Read the model definition and answer for the solid it produces. Units are mm, in the model's axes. Face numbers are marked on the shaded views. Round coordinates to 2 decimals unless told otherwise and drop trailing zeros. Write each loop counter-clockwise with the first axis right and the second up, starting at its lowest first coordinate (ties: lowest second). Pieces come first, ordered by that corner, then holes. Notation, with made-up numbers: (-25, 56) - (25, 56) arc R21 ccw to (25, 81) - close; hole circle Ø2 at (19, -23). An arc over 180 degrees is marked (long way). One line per item, written item: value. Start each with the question number.
(1) A cutting plane is placed at A-A, the plane z = 41. Determine the outline of the cut face in (x, y) (3 decimals), plus the area to 3 significant figures.
(2) A cutting plane is placed at B-B, the plane x = 43. Determine the outline of the cut face in (y, z).
(3) Find the intervals of material crossed by L1, parallel to X at y = 0.5, z = 98; L2, parallel to X at y = -5, z = 156; L3, parallel to Z at x = -15, y = -12.5, in increasing order.
(4) Flat-ended cylindrical pins translate along their axes: pin 1 Ø23 at (y, z) = (42, 34.5) entering from -X; pin 2 Ø1.5 at (y, z) = (-16, 246) entering from -X; pin 3 Ø3 at (y, z) = (-24.5, 159.5) entering from -X. Find the tip coordinate at first contact, or state that the pin passes through.
(5) A cutting plane is placed at D-D, the plane z = 225.5. Determine the outline of the cut face in (x, y).
(6) The mould has two halves that part along X. Classify the marked faces 1, 2 and 3: +X half, -X half, draft (parallel to the pull), parting line (faces both ways), or undercut.
(7) A cutting plane is placed at C-C, the plane y = 45.5. Determine the outline of the cut face in (x, z) (3 decimals), plus the area to 3 significant figures.
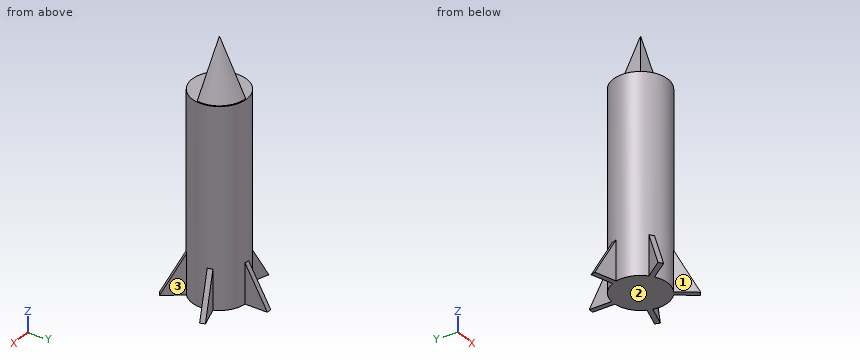
from build123d import *

# Parameters (mm, degrees)
F0_R     = 35.048486
F1_DEPTH = 254
F3_DEPTH = 3.175
F4_COUNT = 5
F6_ANGLE = -100


with BuildPart() as f1:
    # F0 (on Top) → F1 (new body)
    with BuildSketch(Plane.XY):
        Circle(F0_R)
    extrude(amount=F1_DEPTH)

    # F2 (on Right) → F3 (join, symmetric)
    with BuildSketch(Plane.YZ):
        Polygon((0, 114.3), (0, 0), (63.5, 0), align=None)
    extrude(amount=F3_DEPTH, both=True)



with BuildPart() as f4_1:
    # F4: instance of F1
    add(f1.part.rotate(Axis((0, 0, 0), (0, 0, -1)), 1 * 360 / F4_COUNT))


with BuildPart() as f4_2:
    # F4: instance of F1
    add(f1.part.rotate(Axis((0, 0, 0), (0, 0, -1)), 2 * 360 / F4_COUNT))


with BuildPart() as f4_3:
    # F4: instance of F1
    add(f1.part.rotate(Axis((0, 0, 0), (0, 0, -1)), 3 * 360 / F4_COUNT))


with BuildPart() as f4_4:
    # F4: instance of F1
    add(f1.part.rotate(Axis((0, 0, 0), (0, 0, -1)), 4 * 360 / F4_COUNT))


with BuildPart() as f1_1:
    add(f1.part)

    add(f4_1.part)  # F6 merges F4_1

    add(f4_2.part)  # F6 merges F4_2

    add(f4_3.part)  # F6 merges F4_3

    add(f4_4.part)  # F6 merges F4_4
    # F5 (on Right) → F6 (revolve)
    with BuildSketch(Plane.YZ):
        Polygon((0, 320.025444), (0, 253.76758), (34.447256, 252.273053), align=None)
    revolve(axis=Axis((0, 0, 286.896512), (0, 0, 1)), revolution_arc=F6_ANGLE)


solid = f1_1.part
Here are the results:
1. outline: (-39.71, 9.564) - (-34.177, 7.766) arc R35.048 ccw to (-23.085, -26.372) - (-26.505, -31.079) - (-21.367, -34.811) - (-17.948, -30.104) arc R35.048 ccw to (17.948, -30.104) - (21.367, -34.811) - (26.505, -31.079) - (23.085, -26.372) arc R35.048 ccw to (34.177, 7.766) - (39.71, 9.564) - (37.748, 15.603) - (32.215, 13.806) arc R35.048 ccw to (3.175, 34.904) - (3.175, 40.722) - (-3.175, 40.722) - (-3.175, 34.904) arc R35.048 ccw to (-32.215, 13.806) - (-37.748, 15.603) - close
1. area: 4,040 mm²
2. outline: (10.63, 0) - (17.31, 0) - (17.31, 31.06) - (10.63, 34.77) - close
3. L1: -35.04 to 35.04
3. L2: -34.69 to 34.69
3. L3: 0 to 254
4. pin 1: x = -17.27
4. pin 2: x = -31.56
4. pin 3: x = -26.45
5. outline: circle Ø70.1 at (0, 0)
6. face 1: undercut
6. face 2: draft
6. face 3: +X half
7. outline: (-3.175, 0) - (3.175, 0) - (3.175, 32.4) - (-3.175, 32.4) - close
7. area: 206 mm²
